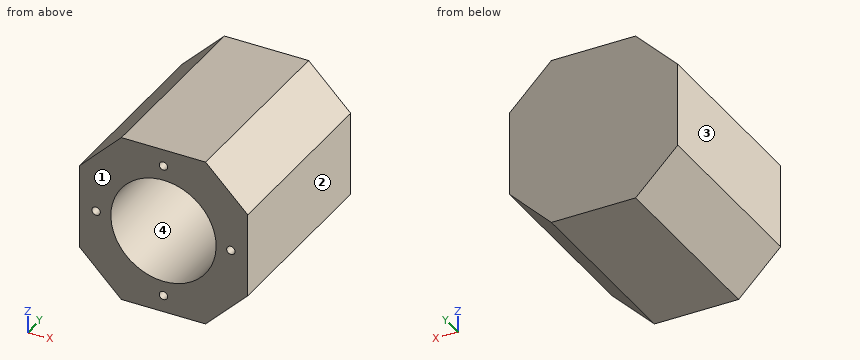
from build123d import *

# Parameters (mm, degrees)
BOSS_EXTRU_1_DEPTH      = 90
ESQUISSE3_R             = 25
ENL_V_MAT_EXTRU_1_DEPTH = 70
ESQUISSE5_R             = 2
ENL_V_MAT_EXTRU_3_DEPTH = 15


with BuildPart() as part:
    # Esquisse2 → Boss.-Extru.1 (new body)
    with BuildSketch(Plane(origin=(0, 0, 0), x_dir=(1, 0, 0), z_dir=(0, 1, 0))):
        Polygon((-20, 40), (-40, 20), (-40, -20), (-20, -40), (20, -40), (40, -20), (40, 20), (20, 40), align=None)
    extrude(amount=BOSS_EXTRU_1_DEPTH)

    # Esquisse3 → Enlèv. mat.-Extru.1 (cut)
    with BuildSketch(Plane.XZ):
        with Locations(Location((0, 0, 0), (0, 0, 270))):
            Circle(ESQUISSE3_R)
    extrude(amount=-ENL_V_MAT_EXTRU_1_DEPTH, mode=Mode.SUBTRACT)

    # Esquisse5 → Enlèv. mat.-Extru.3 (cut)
    with BuildSketch(Plane.XZ):
        with Locations(Location((-32, 0, 0), (0, 0, 270))):
            Circle(ESQUISSE5_R)
        with Locations(Location((0, -32, 0), (0, 0, 270))):
            Circle(ESQUISSE5_R)
        with Locations(Location((32, 0, 0), (0, 0, 270))):
            Circle(ESQUISSE5_R)
        with Locations(Location((0, 32, 0), (0, 0, 270))):
            Circle(ESQUISSE5_R)
    extrude(amount=-ENL_V_MAT_EXTRU_3_DEPTH, mode=Mode.SUBTRACT)


solid = part.part
Here's how the part is built. I have some questions about the finished solid (model axes, mm). Face numbers are marked on the shaded views. Round coordinates to 2 decimals unless told otherwise and drop trailing zeros. Loops run counter-clockwise (first coordinate to the right, second up) from the corner with the lowest first, then second, coordinate; pieces in that order, holes last. Notation, with made-up numbers: (53.5, 78) -> (85.5, 78) arc R26 ccw to (85.5, 105) -> close; hole circle Ø1 at (0, 57). An arc over 180 degrees is marked (long way). Write each question's results on one line, items separated by ' | '.
(1) We'd pull the mould along X, two halves only. Please class the marked faces 1, 2, 3 and 4: released by +X, released by -X, zero draft, split by the parting line, or undercut.
Worked answers:
face 1: zero draft | face 2: released by +X | face 3: released by -X | face 4: undercut
(2) If we section it at D-D, the plane z = -28.5: List the corners of the cut face in (x, y) for me.
Worked answers:
outline: (-31.5, 0) -> (31.5, 0) -> (31.5, 90) -> (-31.5, 90) -> close
(3) If we section it at B-B, the plane z = 32: List the corners of the cut face in (x, y) for me, then the cut area to 3 significant figures.
Worked answers:
outline: (-28, 0) -> (-2, 0) -> (-2, 15) -> (2, 15) -> (2, 0) -> (28, 0) -> (28, 90) -> (-28, 90) -> close | area: 4,980 mm2
(4) For P1, Ø2, axis at x = -27, z = -12.5, coming from the -Y side; P2, Ø15, axis at x = 5, z = 1.5, coming from the -Y side; P3, Ø12, axis at y = 22.5, z = 28, coming from the +X side; P4, Ø2, axis at x = -0.5, z = -32, coming from the -Y side, each with a flat end and sliding along its axis, tell me the tip position at first contact or that it passes through.
Worked answers:
P1: y = 0 | P2: y = 70 | P3: x = 38 | P4: y = 15
(5) If we section it at A-A, the plane y = 66.5: List the corners of the cut face in (x, z) for me.
Worked answers:
outline: (-40, -20) -> (-20, -40) -> (20, -40) -> (40, -20) -> (40, 20) -> (20, 40) -> (-20, 40) -> (-40, 20) -> close; hole circle Ø50 at (0, 0)
(6) If we section it at C-C, the plane x = 32: List the corners of the cut face in (y, z) for me, then the cut area to 3 significant figures.
Worked answers:
outline: (0, -28) -> (90, -28) -> (90, 28) -> (0, 28) -> (0, 2) -> (15, 2) -> (15, -2) -> (0, -2) -> close | area: 4,980 mm2
(7) If I drill on L1, parallel to X at y = 8, z = 0; L2, parallel to X at y = 23, z = 0; L3, parallel to Y at x = 15.5, z = 12.5, over which ranges is the centre line in solid material (lowest first)?
Worked answers:
L1: -40 to -34, -30 to -25, 25 to 30, 34 to 40 | L2: -40 to -25, 25 to 40 | L3: 70 to 90
